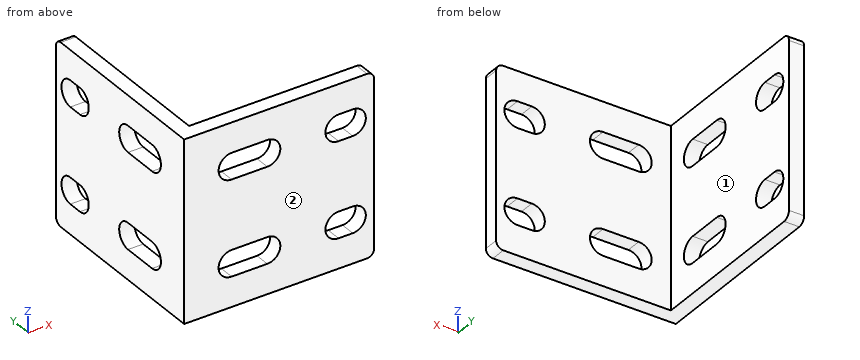
Autodesk Inventor part; units mm, degrees
ref_plane "to_cbm_1_1_XY" through (3.2, 17.5, -10) normal (1, 0, 0) x (0, 0, -1)
ref_plane "to_cbm_1_1_YZ" through (3.2, 17.5, -10) normal (0, 0, -1) x (0, 1, 0)
ref_plane "to_cbm_1_1_ZX" through (3.2, 17.5, -10) normal (0, 1, 0) x (1, 0, 0)
sketch "Sketch_1" plane through (0, 0, 0) normal (1, 0, 0) x (0, 1, 0)
  line L0 (38.5, 19) -> (0, 19)
  line L1 (0, 19) -> (0, -19)
  line L2 (0, -19) -> (38.5, -19)
  arc A0 (38.5, -19) -> (40, -17.5) centre (38.5, -17.5) ccw
  line L3 (40, -17.5) -> (40, 17.5)
  arc A1 (40, 17.5) -> (38.5, 19) centre (38.5, 17.5) ccw
  line L4 (17.5, -7.25) -> (10, -7.25)
  arc A2 (10, -7.25) -> (10, -12.75) centre (10, -10) ccw
  line L5 (10, -12.75) -> (17.5, -12.75)
  arc A3 (17.5, -12.75) -> (17.5, -7.25) centre (17.5, -10) ccw
  line L6 (35.5, -7.25) -> (32.5, -7.25)
  arc A4 (32.5, -7.25) -> (32.5, -12.75) centre (32.5, -10) ccw
  line L7 (32.5, -12.75) -> (35.5, -12.75)
  arc A5 (35.5, -12.75) -> (35.5, -7.25) centre (35.5, -10) ccw
  line L8 (17.5, 12.75) -> (10, 12.75)
  arc A6 (10, 12.75) -> (10, 7.25) centre (10, 10) ccw
  line L9 (10, 7.25) -> (17.5, 7.25)
  arc A7 (17.5, 7.25) -> (17.5, 12.75) centre (17.5, 10) ccw
  line L10 (35.5, 12.75) -> (32.5, 12.75)
  arc A8 (32.5, 12.75) -> (32.5, 7.25) centre (32.5, 10) ccw
  line L11 (32.5, 7.25) -> (35.5, 7.25)
  arc A9 (35.5, 7.25) -> (35.5, 12.75) centre (35.5, 10) ccw
extrude "Extrusion1" add sketch "Sketch_1" along normal blind 3.2
sketch "Sketch_3" plane through (0, 0, 0) normal (0, 1, 0) x (-1, 0, 0)
  line L0 (0, 19) -> (-38.5, 19)
  arc A0 (-38.5, 19) -> (-40, 17.5) centre (-38.5, 17.5) ccw
  line L1 (-40, 17.5) -> (-40, -17.5)
  arc A1 (-40, -17.5) -> (-38.5, -19) centre (-38.5, -17.5) ccw
  line L2 (-38.5, -19) -> (0, -19)
  line L3 (0, -19) -> (0, 19)
  arc A2 (-32.5, -12.75) -> (-32.5, -7.25) centre (-32.5, -10) ccw
  line L4 (-32.5, -7.25) -> (-35.5, -7.25)
  arc A3 (-35.5, -7.25) -> (-35.5, -12.75) centre (-35.5, -10) ccw
  line L5 (-35.5, -12.75) -> (-32.5, -12.75)
  arc A4 (-32.5, 7.25) -> (-32.5, 12.75) centre (-32.5, 10) ccw
  line L6 (-32.5, 12.75) -> (-35.5, 12.75)
  arc A5 (-35.5, 12.75) -> (-35.5, 7.25) centre (-35.5, 10) ccw
  line L7 (-35.5, 7.25) -> (-32.5, 7.25)
  arc A6 (-10, -12.75) -> (-10, -7.25) centre (-10, -10) ccw
  line L8 (-10, -7.25) -> (-17.5, -7.25)
  arc A7 (-17.5, -7.25) -> (-17.5, -12.75) centre (-17.5, -10) ccw
  line L9 (-17.5, -12.75) -> (-10, -12.75)
  arc A8 (-10, 7.25) -> (-10, 12.75) centre (-10, 10) ccw
  line L10 (-10, 12.75) -> (-17.5, 12.75)
  arc A9 (-17.5, 12.75) -> (-17.5, 7.25) centre (-17.5, 10) ccw
  line L11 (-17.5, 7.25) -> (-10, 7.25)
extrude "Extrusion2" add sketch "Sketch_3" along normal blind 3.2
ref_plane "to_cbm_1_1_XY" through (3.2, 17.5, -10) normal (1, 0, 0) x (0, 0, -1)
ref_plane "to_cbm_1_1_YZ" through (3.2, 17.5, -10) normal (0, 0, -1) x (0, 1, 0)
ref_plane "to_cbm_1_1_ZX" through (3.2, 17.5, -10) normal (0, 1, 0) x (1, 0, 0)
ref_plane "to_cbm_1_2_XY" through (3.2, 17.5, 10) normal (1, 0, 0) x (0, 0, -1)
ref_plane "to_cbm_1_2_YZ" through (3.2, 17.5, 10) normal (0, 0, -1) x (0, 1, 0)
ref_plane "to_cbm_1_2_ZX" through (3.2, 17.5, 10) normal (0, 1, 0) x (1, 0, 0)
ref_plane "to_cbm_1_3_XY" through (3.2, 35.5, -10) normal (1, 0, 0) x (0, 0, -1)
ref_plane "to_cbm_1_3_YZ" through (3.2, 35.5, -10) normal (0, 0, -1) x (0, 1, 0)
ref_plane "to_cbm_1_3_ZX" through (3.2, 35.5, -10) normal (0, 1, 0) x (1, 0, 0)
ref_plane "to_cbm_1_4_XY" through (3.2, 35.5, 10) normal (1, 0, 0) x (0, 0, -1)
ref_plane "to_cbm_1_4_YZ" through (3.2, 35.5, 10) normal (0, 0, -1) x (0, 1, 0)
ref_plane "to_cbm_1_4_ZX" through (3.2, 35.5, 10) normal (0, 1, 0) x (1, 0, 0)
ref_plane "to_cbm_2_1_XY" through (17.5, 3.2, 10) normal (0, 1, 0) x (1, 0, 0)
ref_plane "to_cbm_2_1_YZ" through (17.5, 3.2, 10) normal (1, 0, 0) x (0, 0, -1)
ref_plane "to_cbm_2_1_ZX" through (17.5, 3.2, 10) normal (0, 0, -1) x (0, 1, 0)
ref_plane "to_cbm_2_2_XY" through (17.5, 3.2, -10) normal (0, 1, 0) x (1, 0, 0)
ref_plane "to_cbm_2_2_YZ" through (17.5, 3.2, -10) normal (1, 0, 0) x (0, 0, -1)
ref_plane "to_cbm_2_2_ZX" through (17.5, 3.2, -10) normal (0, 0, -1) x (0, 1, 0)
ref_plane "to_cbm_2_3_XY" through (35.5, 3.2, 10) normal (0, 1, 0) x (1, 0, 0)
ref_plane "to_cbm_2_3_YZ" through (35.5, 3.2, 10) normal (1, 0, 0) x (0, 0, -1)
ref_plane "to_cbm_2_3_ZX" through (35.5, 3.2, 10) normal (0, 0, -1) x (0, 1, 0)
ref_plane "to_cbm_2_4_XY" through (35.5, 3.2, -10) normal (0, 1, 0) x (1, 0, 0)
ref_plane "to_cbm_2_4_YZ" through (35.5, 3.2, -10) normal (1, 0, 0) x (0, 0, -1)
ref_plane "to_cbm_2_4_ZX" through (35.5, 3.2, -10) normal (0, 0, -1) x (0, 1, 0)
ref_plane "to_hntp5_1_1_XY" through (-2, 17.5, -10) normal (-1, 0, 0) x (0, -1, 0)
ref_plane "to_hntp5_1_1_YZ" through (-2, 17.5, -10) normal (0, -1, 0) x (0, 0, 1)
ref_plane "to_hntp5_1_1_ZX" through (-2, 17.5, -10) normal (0, 0, 1) x (-1, 0, 0)
ref_plane "to_hntp5_1_2_XY" through (-2, 17.5, 10) normal (-1, 0, 0) x (0, -1, 0)
ref_plane "to_hntp5_1_2_YZ" through (-2, 17.5, 10) normal (0, -1, 0) x (0, 0, 1)
ref_plane "to_hntp5_1_2_ZX" through (-2, 17.5, 10) normal (0, 0, 1) x (-1, 0, 0)
ref_plane "to_hntp5_1_3_XY" through (-2, 35.5, -10) normal (-1, 0, 0) x (0, -1, 0)
ref_plane "to_hntp5_1_3_YZ" through (-2, 35.5, -10) normal (0, -1, 0) x (0, 0, 1)
ref_plane "to_hntp5_1_3_ZX" through (-2, 35.5, -10) normal (0, 0, 1) x (-1, 0, 0)
ref_plane "to_hntp5_1_4_XY" through (-2, 35.5, 10) normal (-1, 0, 0) x (0, -1, 0)
ref_plane "to_hntp5_1_4_YZ" through (-2, 35.5, 10) normal (0, -1, 0) x (0, 0, 1)
ref_plane "to_hntp5_1_4_ZX" through (-2, 35.5, 10) normal (0, 0, 1) x (-1, 0, 0)
ref_plane "to_hntp5_2_1_XY" through (17.5, -2, 10) normal (0, -1, 0) x (-1, 0, 0)
ref_plane "to_hntp5_2_1_YZ" through (17.5, -2, 10) normal (-1, 0, 0) x (0, 0, -1)
ref_plane "to_hntp5_2_1_ZX" through (17.5, -2, 10) normal (0, 0, -1) x (0, -1, 0)
ref_plane "to_hntp5_2_2_XY" through (17.5, -2, -10) normal (0, -1, 0) x (-1, 0, 0)
ref_plane "to_hntp5_2_2_YZ" through (17.5, -2, -10) normal (-1, 0, 0) x (0, 0, -1)
ref_plane "to_hntp5_2_2_ZX" through (17.5, -2, -10) normal (0, 0, -1) x (0, -1, 0)
ref_plane "to_hntp5_2_3_XY" through (35.5, -2, 10) normal (0, -1, 0) x (-1, 0, 0)
ref_plane "to_hntp5_2_3_YZ" through (35.5, -2, 10) normal (-1, 0, 0) x (0, 0, -1)
ref_plane "to_hntp5_2_3_ZX" through (35.5, -2, 10) normal (0, 0, -1) x (0, -1, 0)
ref_plane "to_hntp5_2_4_XY" through (35.5, -2, -10) normal (0, -1, 0) x (-1, 0, 0)
ref_plane "to_hntp5_2_4_YZ" through (35.5, -2, -10) normal (-1, 0, 0) x (0, 0, -1)
ref_plane "to_hntp5_2_4_ZX" through (35.5, -2, -10) normal (0, 0, -1) x (0, -1, 0)
properties part number "HPTBDW5-SEP_b."
Geometry check sheet. Reference: the model listing, model coordinates, mm. Face numbers are marked on the shaded views. A direction names the side the tool comes from. Round coordinates to 2 decimals unless told otherwise and drop trailing zeros. Order: outer loops, then holes, each group sorted by start corner. A loop starts at its lowest first (then second) coordinate and runs counter-clockwise, first axis right, second up. Notation, with made-up numbers: M 46,58 L 53,58 A11 ccw 53,74 Z; hole C -3,72 d9. An arc over 180 degrees is marked long. Answer in a Markdown table with one row per item.
(1) Tool access check on the marked faces 1 and 2. Record the directions out of +Z, -Z, +X, -X, +Y, -Y that give a thin tool (end or side, any length) a straight path to the whole face; none if there is none.
Responses:
| item | result |
|---|---|
| face 1 | +Z, -Z, +X, +Y |
| face 2 | +Z, -Z, +X, -X, -Y |
(2) Sectioned sample at B-B, the plane z = -10. Record the cut outline in (x, y), and give its area (3 significant figures).
Responses:
| item | result |
|---|---|
| outline | M 0,0 L 7.25,0 L 7.25,3.2 L 3.2,3.2 L 3.2,7.25 L 0,7.25 Z; M 0,20.25 L 3.2,20.25 L 3.2,29.75 L 0,29.75 Z; M 0,38.25 L 3.2,38.25 L 3.2,40 L 0,40 Z; M 20.25,0 L 29.75,0 L 29.75,3.2 L 20.25,3.2 Z; M 38.25,0 L 40,0 L 40,3.2 L 38.25,3.2 Z |
| area | 108 mm² |
(3) Scan lines: probe 1 along Z at (x, y) = (3, 16.5); probe 2 along X at (y, z) = (4, 16). Record each from-to range of solid material in increasing order. Write a range as from..to.
Responses:
| item | result |
|---|---|
| probe 1 | z = -19..-12.75, -7.25..7.25, 12.75..19 |
| probe 2 | x = 0..3.2 |
(4) Sectioned sample at C-C, the plane y = 8.5. Record the cut outline in (x, z), and give its area (3 significant figures).
Responses:
| item | result |
|---|---|
| outline | M 0,-19 L 3.2,-19 L 3.2,-12.3 L 0,-12.3 Z; M 0,-7.7 L 3.2,-7.7 L 3.2,7.7 L 0,7.7 Z; M 0,12.3 L 3.2,12.3 L 3.2,19 L 0,19 Z |
| area | 92.1 mm² |
(5) Sectioned sample at D-D, the plane z = -3. Record the cut outline in (x, y).
Responses:
| item | result |
|---|---|
| outline | M 0,0 L 40,0 L 40,3.2 L 3.2,3.2 L 3.2,40 L 0,40 Z |
(6) Sectioned sample at A-A, the plane x = 15. Record the cut outline in (y, z).
Responses:
| item | result |
|---|---|
| outline | M 0,-19 L 3.2,-19 L 3.2,-12.75 L 0,-12.75 Z; M 0,-7.25 L 3.2,-7.25 L 3.2,7.25 L 0,7.25 Z; M 0,12.75 L 3.2,12.75 L 3.2,19 L 0,19 Z |
(7) Go/stop test with flat-tipped pins: P1, Ø1, axis at y = 8, z = -12.5, coming from the +X side; P2, Ø5, axis at x = 6, z = 2.5, coming from the +Y side. Record where each tip stops, or that it passes through.
Responses:
| item | result |
|---|---|
| P1 | stops at x = 3.2 |
| P2 | stops at y = 3.2 |
